from build123d import *

# Parameters (mm, degrees)
SKETCH1_R                = 31
BOSS_EXTRUDE1_DEPTH      = 5
BOSS_EXTRUDE2_DEPTH      = 30
BOSS_EXTRUDE2_DEPTH_BACK = 5
SKETCH2_W                = 140
SKETCH2_H                = 87.5
SKETCH2_W_2              = 120
SKETCH2_H_2              = 67.5
BOSS_EXTRUDE3_START      = -6.5
BOSS_EXTRUDE3_OUTLINE_R  = 100
BOSS_EXTRUDE3_OUTLINE_W  = 140
BOSS_EXTRUDE3_OUTLINE_H  = 87.5
BOSS_EXTRUDE3_DEPTH      = 16.196699026
SKETCH4_W                = 7
SKETCH4_H                = 2
FILLET1_R                = 5
SKETCH5_R                = 1.5
CUT_EXTRUDE1_DEPTH       = 10


# Read off the part's stored shape, not the designer's step: Boss-Extrude3
with BuildPart() as part:
    # Sketch1 → Boss-Extrude1 (new body)
    with BuildSketch(Plane.XY):
        Polygon((41.5, 33.75), (-78.5, 33.75), (-78.5, 28.75), (-43.5, 28.75), (-43.5, -33.75), (41.5, -33.75), align=None)
        Circle(SKETCH1_R, mode=Mode.SUBTRACT)
    extrude(amount=-BOSS_EXTRUDE1_DEPTH)

    # Sketch2 → Boss-Extrude2 (add, two sides: drawn at the far end of the back side and taken through both)
    with BuildSketch(Plane(origin=(0, 0, -5), x_dir=(-1, 0, 0), z_dir=(0, 0, -1)).offset(-BOSS_EXTRUDE2_DEPTH_BACK)):
        with Locations((18.5, 0)):
            Rectangle(SKETCH2_W, SKETCH2_H)
        with Locations((18.5, 0)):
            Rectangle(SKETCH2_W_2, SKETCH2_H_2, mode=Mode.SUBTRACT)
    extrude(amount=BOSS_EXTRUDE2_DEPTH + BOSS_EXTRUDE2_DEPTH_BACK)

    # Boss-Extrude3 outline → Boss-Extrude3 (add)
    with BuildSketch(Plane.XY.offset(-15).offset(BOSS_EXTRUDE3_START)):
        Circle(BOSS_EXTRUDE3_OUTLINE_R)
        with Locations((-18.5, 0)):
            Rectangle(BOSS_EXTRUDE3_OUTLINE_W, BOSS_EXTRUDE3_OUTLINE_H, mode=Mode.SUBTRACT)
    extrude(amount=BOSS_EXTRUDE3_DEPTH)

    # Sketch4 → Cut-Revolve1 (revolve, cut)
    with BuildSketch(Plane(origin=(0, 0, 0), x_dir=(0, 0, -1), z_dir=(1, 0, 0)), mode=Mode.PRIVATE) as cut_revolve1_sk:
        with Locations((14.5, 99)):
            Rectangle(SKETCH4_W, SKETCH4_H)
    revolve(cut_revolve1_sk.sketch.rotate(Axis((0, 0, 0), (0, 0, -1)), 90), axis=Axis((0, 0, 0), (0, 0, -1)), mode=Mode.SUBTRACT)

    # Fillet1
    fillet1_edges = [part.edges().sort_by_distance(p)[0] for p in [
        (-88.5, -43.75, -28.25),
        (51.5, -43.75, -28.25),
        (-88.5, 43.75, -28.25),
        (51.5, 43.75, -28.25),
    ]]
    fillet(fillet1_edges, radius=FILLET1_R)

    # Sketch5 → Cut-Extrude1 (cut)
    with BuildSketch(Plane(origin=(0, 0, -35), x_dir=(-1, 0, 0), z_dir=(0, 0, -1))):
        with Locations((-46.5, 38.75)):
            Circle(SKETCH5_R)
        with Locations((-46.5, -38.75)):
            Circle(SKETCH5_R)
        with Locations((83.5, -38.75)):
            Circle(SKETCH5_R)
        with Locations((83.5, 38.75)):
            Circle(SKETCH5_R)
    extrude(amount=-CUT_EXTRUDE1_DEPTH, mode=Mode.SUBTRACT)


solid = part.part
For this review, take the finished solid that the model builds, in its own axes (mm). A direction names the side the tool comes from. Round coordinates to 2 decimals unless told otherwise and drop trailing zeros. Loops run counter-clockwise (first coordinate to the right, second up) from the corner with the lowest first, then second, coordinate; pieces in that order, holes last. Notation, with made-up numbers: (-4.75, -14.75) - (49.25, -14.75) arc R7 ccw to (49.25, -1.75) - close; hole circle Ø3 at (62, 58.25). An arc over 180 degrees is marked (long way). Put each result on its own line as item: value. Start each with the question number.
1. Consider section A-A on x = 0. State the section outline as (y, z) points, plus the area to 3 significant figures.
2. Consider section D-D on y = -72. State the section outline as (x, z) points.
3. Consider section B-B on z = -31.5. State the section outline as (x, y) points, plus the area to 3 significant figures.
4. Consider section C-C on z = -15.5. State the section outline as (x, y) points, plus the area to 3 significant figures.
5. Mouldability with a two-part tool opening along X and no side actions: class faces 4 (the flat face through (-43.5, -2, -2)), 5 (the cylindrical face through (-87, -42.32, -28.34)), 6 (the flat face through (-18, -43.75, -28)), 7 (the flat face through (41.5, 0, -20)) as +X half, -X half, draft (parallel to the pull), parting line (faces both ways), or undercut.
6. Insertion check: P1, Ø1.5, axis at x = -9.5, z = -29.5, coming from the -Y side; P2, Ø4, axis at y = 42.5, z = -11, coming from the +X side; P3, Ø1.8, axis at x = 46.5, y = -38.75, coming from the -Z side. Each pin has a flat end and moves straight along its axis. Give the tip position at first contact, or say it passes through.
7. For faces 1 (the flat face through (-32, 0, -5)), 2 (the flat face through (-74, 66, -11)), 3 (the cylindrical face through (-87, 42.32, -28.34)), list the 3-axis set-ups (+Z, -Z, +X, -X, +Y, -Y) from which the entire face can be reached by the end or side of a thin tool; tool diameter is ignored.
8. For probe 1 along Y at (x, z) = (46.5, -27.25); probe 2 along X at (y, z) = (38, -30); probe 3 along X at (y, z) = (-21, -27), list the stretches that pass through material, from the lowest coordinate up. Write a range as [from, to].
Result sheet:
1. outline: (-100, -21.5) - (-43.75, -21.5) - (-43.75, -35) - (-33.75, -35) - (-33.75, -5) - (-31, -5) - (-31, 0) - (-43.75, 0) - (-43.75, -5.3) - (-100, -5.3) - (-100, -11) - (-98, -11) - (-98, -18) - (-100, -18) - close; (31, -5) - (33.75, -5) - (33.75, -35) - (43.75, -35) - (43.75, -21.5) - (100, -21.5) - (100, -18) - (98, -18) - (98, -11) - (100, -11) - (100, -5.3) - (43.75, -5.3) - (43.75, 0) - (31, 0) - close
1. area: 2,520 mm^2
2. outline: (-69.4, -21.5) - (69.4, -21.5) - (69.4, -18) - (66.48, -18) - (66.48, -11) - (69.4, -11) - (69.4, -5.3) - (-69.4, -5.3) - (-69.4, -11) - (-66.48, -11) - (-66.48, -18) - (-69.4, -18) - close
3. outline: (-88.5, -38.75) arc R5 ccw to (-83.5, -43.75) - (46.5, -43.75) arc R5 ccw to (51.5, -38.75) - (51.5, 38.75) arc R5 ccw to (46.5, 43.75) - (-83.5, 43.75) arc R5 ccw to (-88.5, 38.75) - close; hole circle Ø3 at (-83.5, -38.75); hole circle Ø3 at (-83.5, 38.75); hole (-78.5, -33.75) - (41.5, -33.75) - (41.5, 33.75) - (-78.5, 33.75) - close; hole circle Ø3 at (46.5, -38.75); hole circle Ø3 at (46.5, 38.75)
3. area: 4,100 mm^2
4. outline: circle Ø196 at (0, 0); hole (-78.5, -33.75) - (41.5, -33.75) - (41.5, 33.75) - (-78.5, 33.75) - close
4. area: 22,100 mm^2
5. face 4: undercut
5. face 5: -X half
5. face 6: draft
5. face 7: undercut
6. P1: y = -43.75
6. P2: x = 91.43
6. P3: z = -25
7. face 1: -Z
7. face 2: none
7. face 3: -Z, -X, +Y
8. probe 1: [-43.75, -40.25], [-37.25, 37.25], [40.25, 43.75]
8. probe 2: [-88.5, -84.8], [-82.2, 45.2], [47.8, 51.5]
8. probe 3: [-88.5, -78.5], [41.5, 51.5]
